Can you work these out from the model? Positions are in its coordinate system, mm. A direction names the side the tool comes from. Coordinates: 2 decimals unless noted, no trailing zeros. Order: outer loops, then holes, each group sorted by start corner. A loop starts at its lowest first (then second) coordinate and runs counter-clockwise, first axis right, second up. Notation, with made-up numbers: (69, 41.5) - (89, 41.5) arc R20 ccw to (89, 69.5) - close; hole circle Ø11 at (55, -28.75). An arc over 180 degrees is marked (long way). Use a Markdown table: item, result. Add a question column.
(1) I want a section at A-A (y = 6.35). State how many separate pieces and enclosed holes the cut face has, and give its area (3 significant figures).
(2) We'd pull the mould along Z, two halves only. Please class faces 1 (the flat face through (-1, 9, 6.35)), 2 (the cylindrical face through (103.616, 6.267, 0.836)), 3 (the flat face through (-87.984, 6.267, -10.197)): pulls with the +Z half, pulls with the -Z half, needs draft (parallel to the pull), parting line crosses it, or undercut.
(3) For pin 1 Ø5 at (x, z) = (-101.6, -12.7) entering from +Y; pin 2 Ø1.5 at (x, y) = (72, 2) entering from -Z; pin 3 Ø4 at (x, z) = (-101.6, 0) entering from -Y, each with a flat end and sliding along its axis, tell me the tip position at first contact or that it passes through.
(4) I want a section at D-D (x = 70.5). List the corners of the cut face in (y, z) for me, and give its area (3 significant figures).
(5) On a 3-axis mill with a long thin cutter (end or side, diameter ignored), from which of +Z, -Z, +X, -X, +Y, -Y can I reach the whole of each face in a straight line? I mean faces 4 (the flat face through (88.23, 6.27, -10.44)), 5 (the flat face through (88.31, 12.499, -10.245)), 6 (the cylindrical face through (103.616, 6.267, -11.864)), 7 (the flat face through (-88.063, 0.201, -9.999)), 8 (the cylindrical face through (-0.47, 4.22, 2.43)). Say none if no direction works.
(6) I want a section at C-C (z = -6.5). List the corners of the cut face in (x, y) for me.
(7) If I drill on L1, parallel to Z at x = -101.6, y = 4.5; L2, parallel to X at y = 9.75, z = 0, over which ranges is the centre line in solid material (lowest first)? Write a range as [from, to].
(8) I want a section at B-B (x = 0). List the corners of the cut face in (y, z) for me.
```python
from build123d import *

# Parameters (mm, degrees)
SKETCH1_R               = 2.1828125
BOSS_EXTRUDE1_DEPTH     = 12.7
CHAMFER1_SIZE           = 1.5875
SKETCH2_R               = 2.1828125
CUT_EXTRUDE1_DEPTH      = 1
CUT_EXTRUDE1_DEPTH_BACK = 26.4
CHAMFER2_SIZE           = 0.396875


with BuildPart() as part:
    # Sketch1 → Boss-Extrude1 (new body)
    with BuildSketch(Plane(origin=(0, 0, 0), x_dir=(1, 0, 0), z_dir=(0, 1, 0))):
        Polygon((-106.3625, -6.35), (106.3625, -6.35), (106.3625, 19.05), (96.8375, 19.05), (79.375, 1.5875), (-79.375, 1.5875), (-96.8375, 19.05), (-106.3625, 19.05), align=None)
        with Locations((-101.6, 0)):
            Circle(SKETCH1_R, mode=Mode.SUBTRACT)
        with Locations((-101.6, 12.7)):
            Circle(SKETCH1_R, mode=Mode.SUBTRACT)
        with Locations((101.6, 0)):
            Circle(SKETCH1_R, mode=Mode.SUBTRACT)
        with Locations((101.6, 12.7)):
            Circle(SKETCH1_R, mode=Mode.SUBTRACT)
    extrude(amount=BOSS_EXTRUDE1_DEPTH)

    # Chamfer1
    chamfer1_edges = [part.edges().sort_by_distance(p)[0] for p in [
        (106.3625, 6.35, -19.05),
        (106.3625, 6.35, 6.35),
        (-106.3625, 6.35, 6.35),
        (-106.3625, 6.35, -19.05),
    ]]
    chamfer(chamfer1_edges, length=CHAMFER1_SIZE)

    # Sketch2 → Cut-Extrude1 (cut, two sides)
    with BuildSketch(Plane.XY.offset(6.35)) as cut_extrude1_sk:
        with Locations((0, 6.35)):
            Circle(SKETCH2_R)
    extrude(amount=CUT_EXTRUDE1_DEPTH, mode=Mode.SUBTRACT)
    extrude(cut_extrude1_sk.sketch, amount=-CUT_EXTRUDE1_DEPTH_BACK, mode=Mode.SUBTRACT)

    # Chamfer2
    chamfer2_edges = [part.edges().sort_by_distance(p)[0] for p in [
        (-88.10625, 0, -10.31875),
        (0, 0, -1.5875),
        (88.10625, 0, -10.31875),
        (0, 12.7, -1.5875),
        (-88.10625, 12.7, -10.31875),
        (-100.80625, 12.7, -19.05),
        (-103.7828125, 0, 0),
        (-103.7828125, 12.7, 0),
        (-103.7828125, 0, -12.7),
        (-103.7828125, 12.7, -12.7),
        (99.4171875, 0, 0),
        (99.4171875, 12.7, 0),
        (99.4171875, 0, -12.7),
        (99.4171875, 12.7, -12.7),
        (100.80625, 0, -19.05),
        (100.80625, 12.7, -19.05),
        (106.3625, 0, -6.35),
        (0, 0, 6.35),
        (-106.3625, 0, -6.35),
        (-105.56875, 0, 5.55625),
        (-105.56875, 0, -18.25625),
        (105.56875, 0, 5.55625),
        (105.56875, 0, -18.25625),
        (106.3625, 12.7, -6.35),
        (-106.3625, 12.7, -6.35),
        (0, 12.7, 6.35),
        (-105.56875, 12.7, 5.55625),
        (-105.56875, 12.7, -18.25625),
        (105.56875, 12.7, 5.55625),
        (105.56875, 12.7, -18.25625),
        (-2.1828125, 6.35, 6.35),
        (-2.1828125, 6.35, -1.5875),
        (88.10625, 12.7, -10.31875),
        (-100.80625, 0, -19.05),
    ]]
    chamfer(chamfer2_edges, length=CHAMFER2_SIZE)


solid = part.part
```
Answers follow:
| question | item | result |
|---|---|---|
| 1 | separate pieces | 2 |
| 1 | enclosed holes | 4 |
| 1 | area | 2,230 mm² |
| 2 | face 1 | pulls with the +Z half |
| 2 | face 2 | undercut |
| 2 | face 3 | pulls with the -Z half |
| 3 | pin 1 | stops at y = 12.62 |
| 3 | pin 2 | stops at z = -1.59 |
| 3 | pin 3 | passes through |
| 4 | outline | (0, -1.19) - (0.4, -1.59) - (12.3, -1.59) - (12.7, -1.19) - (12.7, 5.95) - (12.3, 6.35) - (0.4, 6.35) - (0, 5.95) - close |
| 4 | area | 100 mm² |
| 5 | face 4 | -Z, +Y, -Y |
| 5 | face 5 | -Z, +Y |
| 5 | face 6 | +Y, -Y |
| 5 | face 7 | -Z, -Y |
| 5 | face 8 | +Z, -Z |
| 6 | outline | (-106.36, 0.4) - (-105.97, 0) - (-84.85, 0) - (-84.29, 0.4) - (-84.29, 12.3) - (-84.85, 12.7) - (-105.97, 12.7) - (-106.36, 12.3) - close; (84.29, 0.4) - (84.85, 0) - (105.97, 0) - (106.36, 0.4) - (106.36, 12.3) - (105.97, 12.7) - (84.85, 12.7) - (84.29, 12.3) - close |
| 7 | L1 | z = [-19.05, -14.88], [-10.52, -2.18], [2.18, 6.35] |
| 7 | L2 | x = [-106.36, -103.78], [-99.42, 99.42], [103.78, 106.36] |
| 8 | outline | (0, -1.19) - (0.4, -1.59) - (3.77, -1.59) - (4.17, -1.19) - (4.17, 5.95) - (3.77, 6.35) - (0.4, 6.35) - (0, 5.95) - close; (8.53, -1.19) - (8.93, -1.59) - (12.3, -1.59) - (12.7, -1.19) - (12.7, 5.95) - (12.3, 6.35) - (8.93, 6.35) - (8.53, 5.95) - close |
